Read the model definition and answer for the solid it produces. Units are mm, in the model's axes. Face numbers are marked on the shaded views. A direction names the side the tool comes from. Round coordinates to 2 decimals unless told otherwise and drop trailing zeros. Loops run counter-clockwise (first coordinate to the right, second up) from the corner with the lowest first, then second, coordinate; pieces in that order, holes last. Notation, with made-up numbers: M 72.25,2.5 L 81.25,2.5 A30 cw 81.25,29.5 Z; hole C -20.75,-36 d6. An arc over 180 degrees is marked long. Write each question's results on one line, items separated by ' | '.
from build123d import *

# Parameters (mm, degrees)
F0_W     = 50
F0_H     = 50
F1_DEPTH = 10
F2_W     = 8.0474452116
F2_H     = 30
F2_W_2   = 8
F3_DEPTH = 40
F4_R     = 14.99999
F6_D     = 5


# Not quite as in the source:
# - a fillet or chamfer is up to 0.001 mm smaller than in the source, because OpenCascade refuses the exact size


with BuildPart() as f1:
    # F0 (on Top) → F1 (new body)
    with BuildSketch(Plane.XY):
        with Locations((2.2992696613, -1.7406867517)):
            Rectangle(F0_W, F0_H)
    extrude(amount=F1_DEPTH)

    # F2 (on face) → F3 (join)
    with BuildSketch(Plane.XY.offset(10)):
        with Locations((-8.6770077329, -1.7406867517)):
            Rectangle(F2_W, F2_H)
        with Locations((13.2992696613, -1.7406867517)):
            Rectangle(F2_W_2, F2_H)
    extrude(amount=F3_DEPTH)

    # F4 (radius 15 in the source; OpenCascade refuses exactly that, so slightly less here)
    f4_edges = [f1.edges().sort_by_distance(p)[0] for p in [
        (-8.677008, -16.740687, 50),
        (13.29927, -16.740687, 50),
        (-8.677008, 13.259313, 50),
        (13.29927, 13.259313, 50),
    ]]
    fillet(f4_edges, radius=F4_R)

    # F6 (through all)
    with Locations(Plane.YZ.offset(17.2992696613)):
        with Locations((-1.7406867517, 35)):
            Hole(F6_D / 2)


solid = f1.part
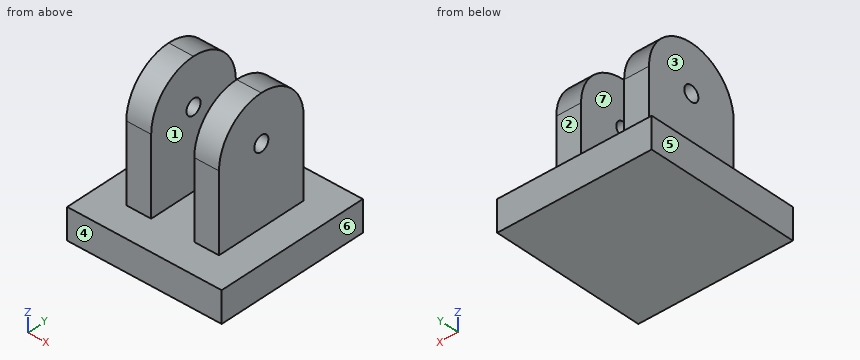
Item 1: Flat-ended cylindrical pins translate along their axes: pin 1 (4 mm diameter, centred on x = 13.5, z = 24, fed in from -Y); pin 2 (3 mm diameter, centred on y = -4.5, z = 39, fed in from -X); pin 3 (6.5 mm diameter, centred on x = 15, z = 25, fed in from +Y); pin 4 (15 mm diameter, centred on x = 11, y = 2, fed in from +Z). Find the tip coordinate at first contact, or state that the pin passes through.
Outcome:
pin 1: stops at y = -16.74 | pin 2: stops at x = -12.7 | pin 3: stops at y = 13.26 | pin 4: stops at z = 50
Item 2: The part is cut by section D-D (y = 17). Determine the outline of the cut face in (x, z), plus the area to 3 significant figures.
Outcome:
outline: M -22.7,0 L 27.3,0 L 27.3,10 L -22.7,10 Z | area: 500 mm2
Item 3: The part is cut by section B-B (z = 16). Determine the outline of the cut face in (x, y), plus the area to 3 significant figures.
Outcome:
outline: M -12.7,-16.74 L -4.65,-16.74 L -4.65,13.26 L -12.7,13.26 Z; M 9.3,-16.74 L 17.3,-16.74 L 17.3,13.26 L 9.3,13.26 Z | area: 481 mm2
Item 4: Straight lines are drawn through the part: line 1 (X direction, y = 11, z = 29); line 2 (Z direction, x = 19, y = -13.5); line 3 (Y direction, x = 14.5, z = 10.5). For each, find the intervals that lie inside material, in ascending order.
Outcome:
line 1: x = -12.7 to -4.65, 9.3 to 17.3 | line 2: z = 0 to 10 | line 3: y = -16.74 to 13.26
Item 5: The part is cut by section C-C (y = -3.5). Determine the outline of the cut face in (x, z), plus the area to 3 significant figures.
Outcome:
outline: M -22.7,0 L 27.3,0 L 27.3,10 L 17.3,10 L 17.3,33.22 L 9.3,33.22 L 9.3,10 L -4.65,10 L -4.65,33.22 L -12.7,33.22 L -12.7,10 L -22.7,10 Z; M -12.7,36.78 L -4.65,36.78 L -4.65,49.9 L -12.7,49.9 Z; M 9.3,36.78 L 17.3,36.78 L 17.3,49.9 L 9.3,49.9 Z | area: 1,080 mm2
Item 6: For the marked faces 1, 2 and 3, determine the directions among +Z, -Z, +X, -X, +Y, -Y from which every point of the face is accessible in a straight line to the end or side of a thin tool.
Outcome:
face 1: +Z, +Y, -Y | face 2: +Z, +X, -X, +Y | face 3: +Z, -X, +Y, -Y
Item 7: The mould has two halves that part along X. Classify the marked faces 4, 5, 6 and 7: pulls with the +X half, pulls with the -X half, needs draft (parallel to the pull), parting line crosses it, or undercut.
Outcome:
face 4: needs draft | face 5: pulls with the -X half | face 6: pulls with the +X half | face 7: undercut
